```python
from build123d import *

# Parameters (mm, degrees)
SKETCH_1_W          = 40.5
SKETCH_1_H          = 20.2
EXTRUDE_1_DEPTH     = 41
SKETCH_2_W          = 56
SKETCH_2_H          = 20.2
EXTRUDE_2_DEPTH     = 2.6
SKETCH_3_R          = 1.75
CUT_EXTRUDE_1_DEPTH = 2.6
SKETCH_4_R          = 2
EXTRUDE_3_DEPTH     = 4


# Read off the part's stored shape, not the designer's step: M3 螺纹孔1
with BuildPart() as part:
    # 草图1 → 凸台-拉伸1 (new body)
    with BuildSketch(Plane.XY):
        Rectangle(SKETCH_1_W, SKETCH_1_H)
    extrude(amount=EXTRUDE_1_DEPTH)

    # 草图2 → 凸台-拉伸2 (add)
    with BuildSketch(Plane.XY.offset(13.3)):
        Rectangle(SKETCH_2_W, SKETCH_2_H)
    extrude(amount=-EXTRUDE_2_DEPTH)

    # 草图3 → 切除-拉伸1 (cut)
    with BuildSketch(Plane(origin=(0, 0, 10.7), x_dir=(-1, 0, 0), z_dir=(0, 0, -1))):
        with Locations((-24, 5)):
            Circle(SKETCH_3_R)
        with Locations(Location((24, 5, 0), (0, 0, 180))):
            Circle(SKETCH_3_R)
        with Locations((24, -5)):
            Circle(SKETCH_3_R)
        with Locations(Location((-24, -5, 0), (0, 0, 180))):
            Circle(SKETCH_3_R)
    extrude(amount=-CUT_EXTRUDE_1_DEPTH, mode=Mode.SUBTRACT)

    # 草图4 → 凸台-拉伸3 (add)
    with BuildSketch(Plane(origin=(0, 0, 0), x_dir=(-1, 0, 0), z_dir=(0, 0, -1))):
        with Locations((9.75, 0)):
            Circle(SKETCH_4_R)
    extrude(amount=EXTRUDE_3_DEPTH)

    # M3 螺纹孔1 outline → M3 螺纹孔1 (revolve, cut)
    with BuildSketch(Plane(origin=(-9.75, 0, 0), x_dir=(1, 0, 0), z_dir=(0, -1, 0))):
        Polygon((1.25, 0), (0, 0.751075774), (0, -4), (1.25, -4), align=None)
    revolve(axis=Axis((-9.75, 0, 0), (0, 0, 1)), mode=Mode.SUBTRACT)


solid = part.part
```
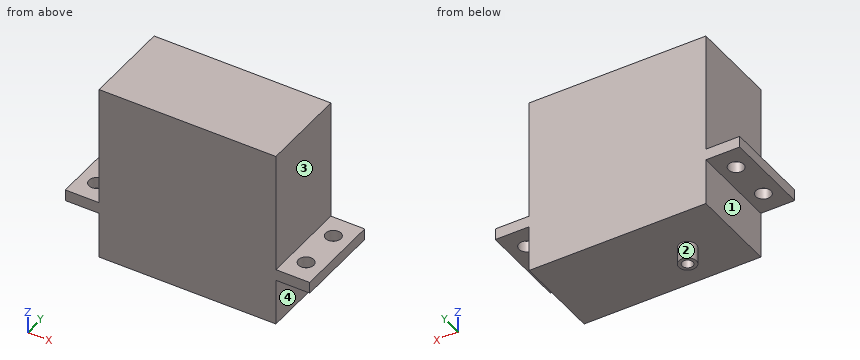
Here's how the part is built. I have some questions about the finished solid (model axes, mm). Face numbers are marked on the shaded views. A direction names the side the tool comes from. Coordinates: 2 decimals unless noted, no trailing zeros. Order: outer loops, then holes, each group sorted by start corner. A loop starts at its lowest first (then second) coordinate and runs counter-clockwise, first axis right, second up.
Item 1: I need wall thicknesses on probe 1 along Y at (x, z) = (-24, 11.55); probe 2 along Y at (x, z) = (-9.75, -1.2); probe 3 along Z at (x, y) = (15.5, 0.75). Which ranges of each line are inside material? Lowest first, please.
Response values:
probe 1: y = -10.1 to -6.75, -3.25 to 3.25, 6.75 to 10.1
probe 2: y = -2 to -1.25, 1.25 to 2
probe 3: z = 0 to 41
Item 2: If we section it at A-A, the plane y = -5: List the corners of the cut face in (x, z) for me.
Response values:
outline: (-28, 10.7) - (-25.75, 10.7) - (-25.75, 13.3) - (-28, 13.3) - close; (-22.25, 10.7) - (-20.25, 10.7) - (-20.25, 0) - (20.25, 0) - (20.25, 10.7) - (22.25, 10.7) - (22.25, 13.3) - (20.25, 13.3) - (20.25, 41) - (-20.25, 41) - (-20.25, 13.3) - (-22.25, 13.3) - close; (25.75, 10.7) - (28, 10.7) - (28, 13.3) - (25.75, 13.3) - close
Item 3: If we section it at D-D, the plane x = -14: List the corners of the cut face in (y, z) for me.
Response values:
outline: (-10.1, 0) - (10.1, 0) - (10.1, 41) - (-10.1, 41) - close
Item 4: If we section it at B-B, the plane x = -24: List the corners of the cut face in (y, z) for me.
Response values:
outline: (-10.1, 10.7) - (-6.75, 10.7) - (-6.75, 13.3) - (-10.1, 13.3) - close; (-3.25, 10.7) - (3.25, 10.7) - (3.25, 13.3) - (-3.25, 13.3) - close; (6.75, 10.7) - (10.1, 10.7) - (10.1, 13.3) - (6.75, 13.3) - close
Item 5: Which directions (+Z, -Z, +X, -X, +Y, -Y) give clear straight access to the entire face, cutting with the end or side of a thin tool? Please do the marked faces 1, 2, 3 and 4.
Response values:
face 1: -Z, -X, +Y, -Y
face 2: -Z
face 3: +Z, +X, +Y, -Y
face 4: -Z, +X, +Y, -Y
Item 6: I'm going to push flat-ended pins straight in: pin 1 Ø8.5 at (x, y) = (22.5, -2) entering from +Z; pin 2 Ø6 at (x, y) = (-20.5, -0.5) entering from -Z; pin 3 Ø5.5 at (x, y) = (-24, 5) entering from +Z; pin 4 Ø8 at (y, z) = (-1, 23) entering from +X. Where does each tip first touch, or does it pass through?
Response values:
pin 1: stops at z = 41
pin 2: stops at z = 0
pin 3: stops at z = 13.3
pin 4: stops at x = 20.25
Item 7: If we section it at C-C, the plane z = 10: List the corners of the cut face in (x, y) for me, then the cut area to 3 significant figures.
Response values:
outline: (-20.25, -10.1) - (20.25, -10.1) - (20.25, 10.1) - (-20.25, 10.1) - close
area: 818 mm2
